Design review of the part built by this model. Coordinates are the model's own, in mm. A direction names the side the tool comes from. Round coordinates to 2 decimals unless told otherwise and drop trailing zeros. Loops run counter-clockwise (first coordinate to the right, second up) from the corner with the lowest first, then second, coordinate; pieces in that order, holes last. Notation, with made-up numbers: M 58,46.5 L 85,46.5 A4 cw 85,51.5 Z; hole C 8,26 d6. An arc over 180 degrees is marked long. Use a Markdown table: item, result.
from build123d import *


with BuildPart() as part:
    # Esboço1 → Revolução1 (revolve)
    with BuildSketch(Plane.XY, mode=Mode.PRIVATE) as revolu_o1_sk:
        Polygon((0, 29), (3, 29), (3, 9), (4, 9), (4, 8), (15, 8), (15, 5.5), (14.25, 5.5), (14.25, 4.5), (15, 4.5), (15, -4.5), (14.25, -4.5), (14.25, -5.5), (15, -5.5), (15, -8), (4, -8), (4, -9), (3, -9), (3, -12), (0, -12), (0, 0), align=None)
    revolve(revolu_o1_sk.sketch.rotate(Axis((0, 0, 0), (0, 1, 0)), 90), axis=Axis((0, 0, 0), (0, 1, 0)))

    # Loft de corte1: read off the stored shape, not the designer's step
    # Loft de corte1: loft between two sections, ruled curve by curve
    loft_de_corte1_from = [
        Edge.make_bspline([(15, 3, -6.499999998), (15, 3, -6.824955331), (15, 2.894080758, -7.511612667), (15, 2.323207443, -8.52324288), (15, 1.314094875, -9.301280201), (15, 0, -9.600009215), (15, -1.314094875, -9.301280201), (15, -2.323207443, -8.52324288), (15, -2.894080758, -7.511612667), (15, -3, -6.824955331), (15, -3, -5.890589586), (15, -3, -4.730897439), (15, -3, -3.107757012), (15, -3, -1.540026122), (15, -3, 0), (15, -3, 1.540026122), (15, -3, 3.107757012), (15, -3, 4.730897439), (15, -3, 5.890589586), (15, -3, 6.824955331), (15, -2.894080758, 7.511612667), (15, -2.323207443, 8.52324288), (15, -1.314094875, 9.301280201), (15, 0, 9.600009215), (15, 1.314094875, 9.301280201), (15, 2.323207443, 8.52324288), (15, 2.894080758, 7.511612667), (15, 3, 6.824955331), (15, 3, 5.890589586), (15, 3, 4.730897439), (15, 3, 3.107757012), (15, 3, 1.540026122), (15, 3, 0), (15, 3, -1.540026122), (15, 3, -3.107757012), (15, 3, -4.730897439), (15, 3, -5.890589586), (15, 3, -6.499999998)], [0, 0, 0, 0, 0.021736358, 0.043472716, 0.065209074, 0.086945432, 0.10868179, 0.130418148, 0.152154506, 0.173890864, 0.173890864, 0.214654506, 0.255418148, 0.29618179, 0.336945432, 0.377709074, 0.418472716, 0.459236358, 0.5, 0.5, 0.521736358, 0.543472716, 0.565209074, 0.586945432, 0.60868179, 0.630418148, 0.652154506, 0.673890864, 0.673890864, 0.714654506, 0.755418148, 0.79618179, 0.836945432, 0.877709074, 0.918472716, 0.959236358, 1, 1, 1, 1], 3),
    ]
    loft_de_corte1_to = [
        Edge.make_bspline([(-15, 1.257174528, -2.723878155), (-15, 1.133171283, -2.781110422), (-15, 0.904058011, -2.868761786), (-15, 0.593969465, -2.944793646), (-15, 0.29436397, -2.990374654), (-15, 0, -3.005552445), (-15, -0.29436397, -2.990374654), (-15, -0.593969465, -2.944793646), (-15, -0.904058011, -2.868761786), (-15, -1.133171283, -2.781110422), (-15, -1.489726085, -2.616546668), (-15, -1.943458979, -2.334486452), (-15, -2.518379121, -1.706139583), (-15, -2.907784722, -0.903903988), (-15, -3.046232987, 0), (-15, -2.907784722, 0.903903988), (-15, -2.518379121, 1.706139583), (-15, -1.943458979, 2.334486452), (-15, -1.489726085, 2.616546668), (-15, -1.133171283, 2.781110422), (-15, -0.904058011, 2.868761786), (-15, -0.593969465, 2.944793646), (-15, -0.29436397, 2.990374654), (-15, 0, 3.005552445), (-15, 0.29436397, 2.990374654), (-15, 0.593969465, 2.944793646), (-15, 0.904058011, 2.868761786), (-15, 1.133171283, 2.781110422), (-15, 1.489726085, 2.616546668), (-15, 1.943458979, 2.334486452), (-15, 2.518379121, 1.706139583), (-15, 2.907784722, 0.903903988), (-15, 3.046232987, 0), (-15, 2.907784722, -0.903903988), (-15, 2.518379121, -1.706139583), (-15, 1.943458979, -2.334486452), (-15, 1.489726085, -2.616546668), (-15, 1.257174528, -2.723878155)], [0, 0, 0, 0, 0.021736358, 0.043472716, 0.065209074, 0.086945432, 0.10868179, 0.130418148, 0.152154506, 0.173890864, 0.173890864, 0.214654506, 0.255418148, 0.29618179, 0.336945432, 0.377709074, 0.418472716, 0.459236358, 0.5, 0.5, 0.521736358, 0.543472716, 0.565209074, 0.586945432, 0.60868179, 0.630418148, 0.652154506, 0.673890864, 0.673890864, 0.714654506, 0.755418148, 0.79618179, 0.836945432, 0.877709074, 0.918472716, 0.959236358, 1, 1, 1, 1], 3),
    ]
    loft_de_corte1 = Solid(Shell([*[Face.make_surface_from_curves(loft_de_corte1_from[k], loft_de_corte1_to[k]) for k in range(1)], Face(Wire(loft_de_corte1_from)), Face(Wire(loft_de_corte1_to))]))
    add(loft_de_corte1, mode=Mode.SUBTRACT)


solid = part.part
1. Take a section at C-C on z = 10. Give the boundary of the cut face in (x, y), and give its area (3 significant figures).
Check values:
| item | result |
|---|---|
| outline | M -11.18,-8 L 11.18,-8 L 11.18,-5.5 L 10.15,-5.5 L 10.15,-4.5 L 11.18,-4.5 L 11.18,4.5 L 10.15,4.5 L 10.15,5.5 L 11.18,5.5 L 11.18,8 L -11.18,8 L -11.18,5.5 L -10.15,5.5 L -10.15,4.5 L -11.18,4.5 L -11.18,-4.5 L -10.15,-4.5 L -10.15,-5.5 L -11.18,-5.5 Z |
| area | 354 mm² |
2. Take a section at D-D on y = 15. Give the boundary of the cut face in (x, z).
Check values:
| item | result |
|---|---|
| outline | C 0,0 d6 |
3. Machinability: for faces 4 (the face through (-0.9, -10.52, -2.86)), 5 (the face through (12, 5.5, -8)), 6 (the face through (-3, 9, 1)), which of the approach directions +Z, -Z, +X, -X, +Y, -Y give a long, thin tool a straight path to every point of the face, cutting with its end or side? Answer none if there is none.
Check values:
| item | result |
|---|---|
| face 4 | -Y |
| face 5 | none |
| face 6 | +Y |
4. The part is to be moulded in two halves that separate along Y. For faces 1 (the face through (3.905, 8.493, 0.867)), 2 (the face through (3, -8, -3)), 3 (the face through (12, 4.5, 8)), say which applies: pulls with the +Y half, pulls with the -Y half, needs draft (parallel to the pull), parting line crosses it, or undercut.
Check values:
| item | result |
|---|---|
| face 1 | needs draft |
| face 2 | pulls with the -Y half |
| face 3 | undercut |
5. Take a section at A-A on z = 13.5. Give the boundary of the cut face in (x, y), and give its area (3 significant figures).
Check values:
| item | result |
|---|---|
| outline | M -6.54,-8 L 6.54,-8 L 6.54,-5.5 L 4.56,-5.5 L 4.56,-4.5 L 6.54,-4.5 L 6.54,4.5 L 4.56,4.5 L 4.56,5.5 L 6.54,5.5 L 6.54,8 L -6.54,8 L -6.54,5.5 L -4.56,5.5 L -4.56,4.5 L -6.54,4.5 L -6.54,-4.5 L -4.56,-4.5 L -4.56,-5.5 L -6.54,-5.5 Z |
| area | 201 mm² |
6. Wall thickness on line 1 along Y through (x, z) = (-3.5, 9); line 2 along Z through (x, y) = (-2, 2); line 3 along Y through (x, z) = (5.5, -5): over which ranges is each line inside the solid? List them lowest first. Write a range as from..to.
Check values:
| item | result |
|---|---|
| line 1 | y = -8..8 |
| line 2 | z = -14.87..-4.39, 4.39..14.87 |
| line 3 | y = -8..-2.5, 2.5..8 |
7. Take a section at B-B on y = 4. Give the boundary of the cut face in (x, z), and give its area (3 significant figures).
Check values:
| item | result |
|---|---|
| outline | C 0,0 d30 |
| area | 707 mm² |
8. Insertion check: pin 1 (3 mm diameter, centred on x = -10.5, z = -9.5, fed in from +Y); pin 2 (10 mm diameter, centred on x = -11, y = 8, fed in from +Z); pin 3 (8 mm diameter, centred on y = -5, z = -8, fed in from -X). Each pin has a flat end and moves straight along its axis. Give the tip position at first contact, or say it passes through.
Check values:
| item | result |
|---|---|
| pin 1 | stops at y = 8 |
| pin 2 | stops at z = 13.75 |
| pin 3 | stops at x = -14.45 |
